Could you check a few things on this drawing? It's one solid part, dimensions in mm from its lowest x, y, z. A direction names the side the tool comes from. Give positions to 0.01 mm unless a question says otherwise; leave off trailing zeros. Loops run counter-clockwise (first coordinate to the right, second up) from the corner with the lowest first, then second, coordinate; pieces in that order, holes last. Notation, with made-up numbers: M -4,51.5 L 37,51.5 A26 ccw 37,73.5 Z; hole C 79.5,30.5 d5. An arc over 180 degrees is marked long. Return JSON: item names as keys, results as strings. Group by question number.
1. If we section it at D-D (z = 31.75): Write out the boundary of the cut face in (x, y) (1 decimal).
2. For pin 1 (12.5 mm diameter, centred on x = 19, z = 16.5, fed in from -Y); pin 2 (3 mm diameter, centred on x = 12.7, z = 31.75, fed in from +Y); pin 3 (2 mm diameter, centred on x = 8, y = 2.5, fed in from +Z) (1 decimal); pin 4 (2 mm diameter, centred on x = 13.5, y = 2, fed in from +Z) (1 decimal), each with a flat end and sliding along its axis, tell me the tip position at first contact or that it passes through.
3. If we section it at A-A (x = 12.7): Write out the boundary of the cut face in (y, z) (1 decimal), plus the area to 3 significant figures.
4. Please list where these lines run through material, in increasing order: line 1 (X direction, y = 4.5, z = 5); line 2 (Z direction, x = 12.7, y = 7.95); line 3 (X direction, y = 0.5, z = 7) (1 decimal).
5. If we mould it in two halves opening along X, with no side actions, what happens to the marked faces 1, 2 and 3? For each: +X half, -X half, draft (parallel to the pull), parting line (faces both ways), or undercut.
6. If we section it at C-C (z = 17): Write out the boundary of the cut face in (x, y) (1 decimal).
7. For the marked faces 4 and 5, which set-ups out of +Z, -Z, +X, -X, +Y, -Y let a thin tool reach every point of the face, with its end or its side?
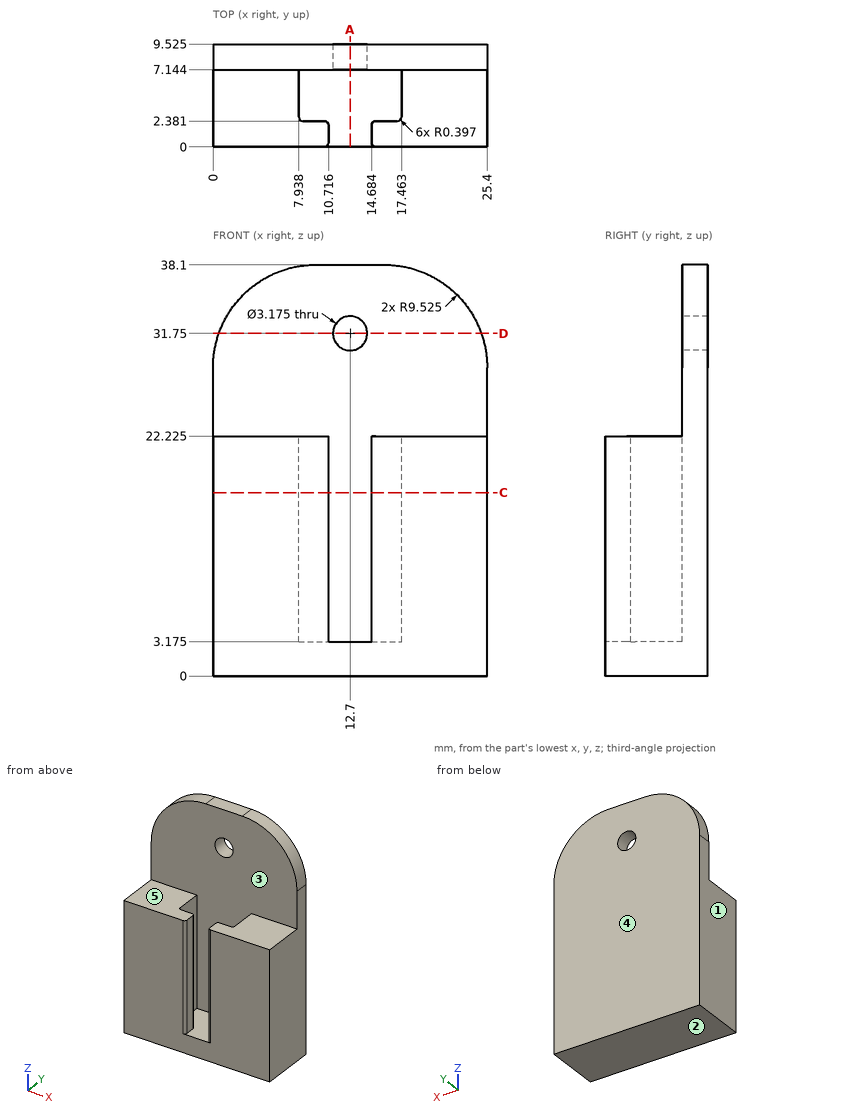
Answer:
{
 "1": {"outline": "M 0.5,7.1 L 11.1,7.1 L 11.1,9.5 L 0.5,9.5 Z; M 14.3,7.1 L 24.9,7.1 L 24.9,9.5 L 14.3,9.5 Z"},
 "2": {"pin 1": "stops at y = 0", "pin 2": "passes through", "pin 3": "stops at z = 22.2", "pin 4": "stops at z = 3.2"},
 "3": {"outline": "M 0,0 L 9.5,0 L 9.5,30.2 L 7.1,30.2 L 7.1,3.2 L 0,3.2 Z; M 7.1,33.3 L 9.5,33.3 L 9.5,38.1 L 7.1,38.1 Z", "area": "106 mm²"},
 "4": {"line 1": "x = 0 to 7.94, 17.46 to 25.4", "line 2": "z = 0 to 30.16, 33.34 to 38.1", "line 3": "x = 0 to 10.7, 14.7 to 25.4"},
 "5": {"face 1": "-X half", "face 2": "draft", "face 3": "undercut"},
 "6": {"outline": "M 0,0 L 10.3,0 A0.4 ccw 10.7,0.4 L 10.7,2 A0.4 ccw 10.3,2.4 L 8.3,2.4 A0.4 cw 7.9,2.8 L 7.9,7.1 L 17.5,7.1 L 17.5,2.8 A0.4 cw 17.1,2.4 L 15.1,2.4 A0.4 ccw 14.7,2 L 14.7,0.4 A0.4 ccw 15.1,0 L 25.4,0 L 25.4,9.5 L 0,9.5 Z"},
 "7": {"face 4": "+Z, -Z, +X, -X, +Y", "face 5": "+Z, +X, -X, -Y"}
}
